Autodesk Inventor part; units mm, degrees
ref_plane "YZ Plane" through (0, 0, 0) normal (1, 0, 0) x (0, 1, 0)
ref_plane "XZ Plane" through (0, 0, 0) normal (0, 1, 0) x (-1, 0, 0)
ref_plane "XY Plane" through (0, 0, 0) normal (0, 0, 1) x (1, 0, 0)
sketch "Szkic1" plane through (0, 0, 0) normal (0, 0, 1) x (1, 0, 0)
  line L0 (0, 0) -> (-32, 0)
  circle A0 centre (-32, 0) radius 2
  circle A1 centre (0, 0) radius 2
  line L1 (-40.5, -6) -> (8.5, -6)
  line L2 (8.5, -6) -> (8.5, 6)
  line L3 (8.5, 6) -> (-40.5, 6)
  line L4 (-40.5, 6) -> (-40.5, -6)
  line L5 (-40.5, -6) -> (8.5, 6) construction
  line L6 (8.5, -6) -> (-40.5, 6) construction
  point P0 (-16, 0)
  dimension "d2" = 32
  dimension "d3" = 4
  dimension "d4" = 4
  dimension "d5" = 49
  dimension "d6" = 12
extrude "Wyciągnięcie proste1" add sketch "Szkic1" along normal blind 5
sketch "Szkic2" plane through (0, 0, 5) normal (0, 0, 1) x (1, 0, 0)
  line L0 (8.5, -6) -> (8.5, 6)
  line L1 (-40.5, -6) -> (8.5, -6)
  line L2 (8.5, 6) -> (4.5, 6)
  line L3 (4.5, 6) -> (4.5, -6)
  line L4 (4.5, -6) -> (8.5, -6)
  line L5 (8.5, -6) -> (8.5, 6)
  line L6 (-40.5, 6) -> (-36.5, 6)
  line L7 (-36.5, 6) -> (-36.5, -6)
  line L8 (-36.5, -6) -> (-40.5, -6)
  line L9 (-40.5, -6) -> (-40.5, 6)
  dimension "d12" = 4
  dimension "d13" = 4
extrude "Wyciągnięcie proste2" add sketch "Szkic2" along normal blind 26
fillet "Zaokrąglenie1" radius 6 4 edges at (-38.5, 6, 31) (-38.5, -6, 31) (6.5, 6, 31) (6.5, -6, 31)
sketch "Szkic3" plane through (-36.5, -6, 5) normal (1, 0, 0) x (0, 0, -1)
  line L0 (0, 5.9057) -> (-21.5, 5.9057)
  circle A0 centre (-21.5, 5.9057) radius 1.5
  point P0 (5, 6)
  dimension "d15" = 21.5
  dimension "d16" = 3
extrude "Wyciągnięcie proste3" cut sketch "Szkic3" along normal mid plane 100
sketch "Szkic4" plane through (0, 0, 5) normal (0, 0, 1) x (1, 0, 0)
  circle A0 centre (0, 0) radius 2
  circle A1 centre (-32, 0) radius 2
  line L0 (4.5, -6) -> (4.5, 6)
  line L1 (4.5, 6) -> (-36.5, 6)
  line L2 (-36.5, 6) -> (-36.5, -6)
  line L3 (-36.5, -6) -> (4.5, -6)
extrude "Wyciągnięcie proste4" cut sketch "Szkic4" against normal blind 1 contours A0 | A1 | L3 L2 L1 L0
properties part number "Zebatka holder"
CAD build for the part. Positions are in the model's coordinates, mm. A direction names the side the tool comes from. Give positions to 0.01 mm unless a question says otherwise; leave off trailing zeros. Order: outer loops, then holes, each group sorted by start corner. A loop starts at its lowest first (then second) coordinate and runs counter-clockwise, first axis right, second up.
(1) Saw through at A-A, the plane z = 8.5. Give the cut face in (x, y).
(2) Flat gauge pin, fed straight in: pin 1 (3.5 mm diameter, centred on x = -32, y = 0, fed in from -Z). Where does the tip first touch, or does it go through?
(3) Saw through at D-D, the plane z = 2. Give the cut face in (x, y), then the cut area to 3 significant figures.
(4) Drill centre lines: L1, parallel to X at y = 0, z = 1.4; L2, parallel to X at y = 0.5, z = 21; L3, parallel to Z at x = -34, y = 5. Where is each one in solid material? Low to high.
(5) Mould opens along Y. For faces 1 (the flat face through (4.5, 0, 18)), 2 (the cylindrical face through (0, 2, 2)), 3 (the cylindrical face through (-38.472, -4.196, 29.289)) say: released by +Y, released by -Y, zero draft, split by the parting line, or undercut.
(6) Tool access for faces 4 (the flat face through (-36.5, 0, 17)), 5 (the flat face through (-16, 6, 1)): list every direction of +Z, -Z, +X, -X, +Y, -Y with a clear straight run to the whole face (end or side of a thin tool).
(7) Saw through at B-B, the plane x = 0. Give the cut face in (y, z), then the cut area to 3 significant figures.
(8) Saw through at C-C, the plane y = 0.5. Give the cut face in (x, z).
Results found:
1. outline: (-40.5, -6) - (-36.5, -6) - (-36.5, 6) - (-40.5, 6) - close; (4.5, -6) - (8.5, -6) - (8.5, 6) - (4.5, 6) - close
2. pin 1: passes through
3. outline: (-40.5, -6) - (8.5, -6) - (8.5, 6) - (-40.5, 6) - close; hole circle Ø4 at (-32, 0); hole circle Ø4 at (0, 0)
3. area: 563 mm2
4. L1: x = -40.5 to -34, -30 to -2, 2 to 8.5
4. L2: x = -40.5 to -36.5, 4.5 to 8.5
4. L3: z = 0 to 4
5. face 1: zero draft
5. face 2: undercut
5. face 3: released by -Y
6. face 4: +Z, +Y, -Y
6. face 5: +Z, -Z, +X, -X, +Y
7. outline: (-6, 0) - (-2, 0) - (-2, 4) - (-6, 4) - close; (2, 0) - (6, 0) - (6, 4) - (2, 4) - close
7. area: 32.0 mm2
8. outline: (-40.5, 0) - (-33.94, 0) - (-33.94, 4) - (-36.5, 4) - (-36.5, 25.12) - (-40.5, 25.12) - close; (-40.5, 27.88) - (-36.5, 27.88) - (-36.5, 30.98) - (-40.5, 30.98) - close; (-30.06, 0) - (-1.94, 0) - (-1.94, 4) - (-30.06, 4) - close; (1.94, 0) - (8.5, 0) - (8.5, 25.12) - (4.5, 25.12) - (4.5, 4) - (1.94, 4) - close; (4.5, 27.88) - (8.5, 27.88) - (8.5, 30.98) - (4.5, 30.98) - close
